Source: CAD feature listing. Evaluate the final solid. Frame: model axes, mm. Face numbers are marked on the shaded views. A direction names the side the tool comes from. Give positions to 0.01 mm unless a question says otherwise; leave off trailing zeros. Order: outer loops, then holes, each group sorted by start corner. A loop starts at its lowest first (then second) coordinate and runs counter-clockwise, first axis right, second up. Notation, with made-up numbers: M 88.25,10.25 L 107.25,10.25 A16 cw 107.25,24.25 Z; hole C -36,-21 d9. An arc over 180 degrees is marked long. Use CSV: the item, a comma, the result in double quotes. Start each with the question number.
Item 1: First-contact query: pin 1 (4 mm diameter, centred on y = 7, z = 4, fed in from +X); pin 2 (3 mm diameter, centred on x = 8.23, z = 3.18, fed in from +Y); pin 3 (1 mm diameter, centred on y = 6.5, z = 3, fed in from -X). Flat tips, straight axial feed; report the tip coordinate or a pass-through.
Item 2: Section query C-C on z = 5.75. Return loops of the section in (x, y), and give its area (3 significant figures).
Item 3: Section query A-A on x = 0. Return loops of the section in (y, z) (1 decimal).
Item 4: Ray query, probe 1 along Y at (x, z) = (0, 3.5); probe 2 along X at (y, z) = (-2.5, 3); probe 3 along Y at (x, z) = (2, 1). Return the intervals inside material, ascending. Write a range as from..to.
Item 5: Section query B-B on y = -2. Count the separate pieces of the cut face and the enclosed holes in it, and give its area (3 significant figures).
Item 6: Pull-direction query (Y, two-part tool) for the marked faces 1, 2 and 3; classes: +Y half, -Y half, draft (parallel to the pull), parting line (faces both ways), or undercut.
Item 7: Access query for the marked faces 4 and 5. Directions: +Z, -Z, +X, -X, +Y, -Y. A direction counts if a zero-diameter tool reaches every point of the face in a straight line with its end or side. Return the directions, or none.
from build123d import *
from build123d.topology import SkipClean

# Parameters (mm, degrees)
BOSS_EXTRUDE1_DEPTH     = 6.985
CUT_EXTRUDE1_DEPTH      = 19.104903341
CUT_EXTRUDE1_DEPTH_BACK = 19.104903341
SKETCH2_R               = 1.143
SKETCH3_R               = 2.286
CUT_EXTRUDE2_DEPTH      = 21.568811653
BOSS_EXTRUDE2_START     = 1.27
BOSS_EXTRUDE2_DEPTH     = 1.27
BOSS_EXTRUDE3_START     = 2.54
SKETCH5_R               = 11.43
SKETCH5_R_2             = 3.1115
BOSS_EXTRUDE3_DEPTH     = 2.54
SKETCH29_R              = 1.778
CUT_EXTRUDE9_DEPTH      = 21.245185396
CHAMFER3_SIZE           = 2.881011164
CHAMFER3_SIZE_2         = 0.508
CHAMFER4_SIZE           = 0.508
FILLET1_R               = 0.5
SKETCH30_R              = 16.901185141
CUT_EXTRUDE10_DEPTH     = 3.81
CHAMFER5_SIZE           = 0.5


with BuildPart() as part:
    # Sketch1 → Boss-Extrude1 (new body)
    with BuildSketch(Plane.XY):
        with BuildLine():
            Line((3.019756985, -0.75), (11.405367158, -0.75))
            ThreePointArc((11.405367158, -0.75), (-11.43, 0), (11.405367158, 0.75))
            Line((11.405367158, 0.75), (3.019756985, 0.75))
            ThreePointArc((3.019756985, 0.75), (-3.1115, 0), (3.019756985, -0.75))
        make_face()
    extrude(amount=BOSS_EXTRUDE1_DEPTH)

    # Sketch2 → Cut-Extrude1 (cut, two sides: drawn at the far end of the back side and taken through both)
    with BuildSketch(Plane.XZ.offset(-0.75).offset(-CUT_EXTRUDE1_DEPTH_BACK)):
        with Locations(Location((8.230367158, 3.175, 0), (0, 0, 270))):
            Circle(SKETCH2_R)
    extrude(amount=CUT_EXTRUDE1_DEPTH + CUT_EXTRUDE1_DEPTH_BACK, mode=Mode.SUBTRACT)

    # Sketch3 → Cut-Extrude2 (cut, through all)
    with BuildSketch(Plane(origin=(0, 4.179, 0), x_dir=(-1, 0, 0), z_dir=(0, -1, 0))):
        with Locations(Location((-8.230367158, -3.175, 0), (0, 0, 90))):
            Circle(SKETCH3_R)
    extrude(amount=-CUT_EXTRUDE2_DEPTH, mode=Mode.SUBTRACT)

    # Sketch4 → Boss-Extrude2 (add)
    with BuildSketch(Plane(origin=(0, 0, 0), x_dir=(-1, 0, 0), z_dir=(0, 0, -1)).offset(BOSS_EXTRUDE2_START)):
        with BuildLine():
            Line((3.1115, 0), (11.43, 0))
            ThreePointArc((11.43, 0), (0.375202204, 11.42384013), (-11.405367158, 0.75))
            Line((-11.405367158, 0.75), (-3.019756985, 0.75))
            ThreePointArc((-3.019756985, 0.75), (0.377795176, 3.088479084), (3.1115, 0))
        make_face()
    extrude(amount=-BOSS_EXTRUDE2_DEPTH)

    # Sketch5 → Boss-Extrude3 (add)
    with SkipClean():  # the faces are left unmerged after this step: merging them gives an invalid solid
        with BuildSketch(Plane(origin=(0, 0, -1.27), x_dir=(-1, 0, 0), z_dir=(0, 0, -1)).offset(BOSS_EXTRUDE3_START)):
            Circle(SKETCH5_R)
            Circle(SKETCH5_R_2, mode=Mode.SUBTRACT)
        extrude(amount=-BOSS_EXTRUDE3_DEPTH)

    # Sketch29 → Cut-Extrude9 (cut, through all)
    with SkipClean():  # the faces are left unmerged after this step: merging them gives an invalid solid
        with BuildSketch(Plane(origin=(0, -3.75, 0), x_dir=(1, 0, 0), z_dir=(0, 1, 0))):
            with Locations(Location((8.230367158, -3.175, 0), (0, 0, 270))):
                Circle(SKETCH29_R)
        extrude(amount=-CUT_EXTRUDE9_DEPTH, mode=Mode.SUBTRACT)

    # Chamfer3
    # the kernel refuses this chamfer: 2.881011164, 0.508 mm, written as the material it adds along each edge
    with BuildSketch(Plane(origin=(8.230367158, -3.75, 3.175), x_dir=(0, 0, 1), z_dir=(-1, 0, 0))) as chamfer3_piece_1_section:
        Polygon((1.778, -CHAMFER3_SIZE), (1.778 - CHAMFER3_SIZE_2, 0), (1.778, 0), align=None)
    chamfer3_piece_1 = revolve(axis=Axis((8.230367158, -3.75, 3.175), (0, 1, 0)), mode=Mode.PRIVATE)
    chamfer3_piece_1 = chamfer3_piece_1 & Plane(origin=(0, 0, 1.63014176), x_dir=(0.9978448956793416, -0.06561679790026252, 0), z_dir=(0, 0, -1)) * Cylinder(11.43, 12, mode=Mode.PRIVATE)
    add(chamfer3_piece_1)

    # Chamfer4
    chamfer4_edges = [part.edges().sort_by_distance(p)[0] for p in [
        (-11.43, 0, 6.985),
    ]]
    chamfer(chamfer4_edges, length=CHAMFER4_SIZE)

    # Fillet1
    # the kernel refuses this fillet: 0.5 mm, written as the material it takes off along each edge
    with BuildSketch(Plane(origin=(-3.1115, 0, -1.27), x_dir=(-1, 0, 0), z_dir=(0, 0, 1))) as fillet1_piece_1:
        with BuildLine():
            CenterArc((0.46522088, -0.5), FILLET1_R, 90, 82.042030685)
            ThreePointArc((-0.029964068, -0.430776686), (-0.007500056, -0.215908776), (0, 0))
            Line((0, 0), (0.46522088, 0))
        make_face()
    extrude(amount=1.27, mode=Mode.SUBTRACT)
    with BuildSketch(Plane(origin=(-11.43, 0, -1.27), x_dir=(0.022878815711235678, 0.9997382456381528, 0), z_dir=(0, 0, 1))) as fillet1_piece_2:
        with BuildLine():
            CenterArc((0.511570319, -0.499869123), FILLET1_R, 88.689026033, 92.621947934)
            Line((0.011701196, -0.511308531), (0, 0))
            ThreePointArc((0, 0), (0.261504864, 0.002991852), (0.523009727, 0))
        make_face()
    extrude(amount=1.27, mode=Mode.SUBTRACT)
    with BuildSketch(Plane(origin=(3.019756985, -0.75, -0.921304177), x_dir=(1, 0, 0), z_dir=(0, 0, 1))) as fillet1_piece_3:
        with BuildLine():
            CenterArc((0.368521671, -0.5), FILLET1_R, 90, 69.75002962)
            ThreePointArc((-0.100574087, -0.326941714), (-0.04579087, -0.164853974), (0, 0))
            Line((0, 0), (0.368521671, 0))
        make_face()
    extrude(amount=8.827608353, mode=Mode.SUBTRACT)
    with BuildSketch(Plane(origin=(3.019756985, 0.75, 7.906304177), x_dir=(1, 0, 0), z_dir=(0, 0, -1))) as fillet1_piece_4:
        with BuildLine():
            CenterArc((0.368521671, -0.5), FILLET1_R, 90, 69.75002962)
            ThreePointArc((-0.100574087, -0.326941714), (-0.04579087, -0.164853974), (0, 0))
            Line((0, 0), (0.368521671, 0))
        make_face()
    extrude(amount=9.176304177, mode=Mode.SUBTRACT)

    # Sketch30 → Cut-Extrude10 (cut)
    with BuildSketch(Plane(origin=(0, 0, -3.81), x_dir=(-1, 0, 0), z_dir=(0, 0, -1))):
        Circle(SKETCH30_R)
    extrude(amount=-CUT_EXTRUDE10_DEPTH, mode=Mode.SUBTRACT)

    # Chamfer5
    chamfer5_edges = [part.edges().sort_by_distance(p)[0] for p in [
        (-11.43, 0, 0),
    ]]
    chamfer(chamfer5_edges, length=CHAMFER5_SIZE)


solid = part.part
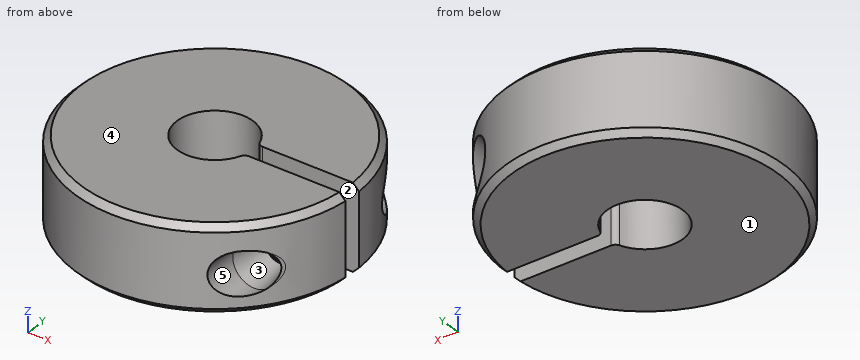
Verdict:
1,pin 1,"x = 10.27"
1,pin 2,"y = 4.18"
1,pin 3,"x = -9.73"
2,outline,"M 2.92,-1.08 A3.11 cw long 2.92,1.08 A0.5 ccw 3.39,0.75 L 11.41,0.75 A11.43 ccw long 11.41,-0.75 L 3.39,-0.75 A0.5 ccw Z"
2,area,"367 mm2"
3,outline,"M -11.4,0.5 L -10.9,0 L -3.1,0 L -3.1,7 L -10.9,7 L -11.4,6.5 Z; M 3.1,0 L 10.9,0 L 11.4,0.5 L 11.4,6.5 L 10.9,7 L 3.1,7 Z"
4,probe 1,"-11.43..-3.11, 3.11..11.43"
4,probe 2,"-11.15..-1.85, 1.85..7.1, 9.36..11.15"
4,probe 3,"-11.25..-2.38, 2.38..11.25"
5,separate pieces,"2"
5,enclosed holes,"1"
5,area,"119 mm2"
6,face 1,"draft"
6,face 2,"undercut"
6,face 3,"-Y half"
7,face 4,"+Z, +X, -X, +Y, -Y"
7,face 5,"-Y"
